```python
from build123d import *

# Parameters (mm, degrees)
PAD_DEPTH       = 30
POCKET_DEPTH    = 28
SKETCH002_R     = 1
POCKET001_DEPTH = 5
SKETCH003_R     = 1.6
POCKET002_DEPTH = 5
POCKET003_DEPTH = 2


with BuildPart() as part:
    # Sketch → Pad (new body)
    with BuildSketch(Plane.XZ):
        Polygon((-68.72, 55.88), (-68.72, -25.12), (-13.72, -25.12), (-13.72, -125.12), (22.28, -125.12), (22.28, -25.12), (77.28, -25.12), (77.28, 55.88), align=None)
    extrude(amount=PAD_DEPTH)

    # Sketch001 (on Face10 of Pad) → Pocket (cut)
    with BuildSketch(Plane.XZ.offset(30)):
        Polygon((-65.72, 52.88), (-65.72, -22.12), (-10.72, -22.12), (-10.72, -122.12), (19.28, -122.12), (19.28, -22.12), (74.28, -22.12), (74.28, 52.88), align=None)
    extrude(amount=-POCKET_DEPTH, mode=Mode.SUBTRACT)

    # Sketch002 (on Face10 of Pad) → Pocket001 (cut)
    with BuildSketch(Plane.XZ.offset(30)):
        with Locations((-11.82, -23.22)):
            Circle(SKETCH002_R)
        with Locations((-11.72, -123.12)):
            Circle(SKETCH002_R)
        with Locations((20.38, -23.22)):
            Circle(SKETCH002_R)
        with Locations((20.28, -123.12)):
            Circle(SKETCH002_R)
        with Locations((-66.72, -23.12)):
            Circle(SKETCH002_R)
        with Locations((75.28, -23.12)):
            Circle(SKETCH002_R)
        with Locations((75.28, 53.88)):
            Circle(SKETCH002_R)
        with Locations((-66.72, 53.88)):
            Circle(SKETCH002_R)
    extrude(amount=-POCKET001_DEPTH, mode=Mode.SUBTRACT)

    # Sketch003 (on Face28 of Pocket001) → Pocket002 (cut)
    with BuildSketch(Plane.XZ.offset(2)):
        with Locations((-7.62, -119.62)):
            Circle(SKETCH003_R)
        with Locations((16.78, -119.62)):
            Circle(SKETCH003_R)
        with Locations((-7.62, -26.62)):
            Circle(SKETCH003_R)
        with Locations((16.78, -26.62)):
            Circle(SKETCH003_R)
    extrude(amount=-POCKET002_DEPTH, mode=Mode.SUBTRACT)

    # Sketch004 (on Face5 of Pocket002) → Pocket003 (cut)
    with BuildSketch(Plane.XZ.offset(30)):
        Polygon((-67.97, 55.13), (-67.97, -24.37), (-12.97, -24.37), (-12.97, -124.37), (21.53, -124.37), (21.53, -24.37), (76.53, -24.37), (76.53, 55.13), align=None)
    extrude(amount=-POCKET003_DEPTH, mode=Mode.SUBTRACT)


solid = part.part
```
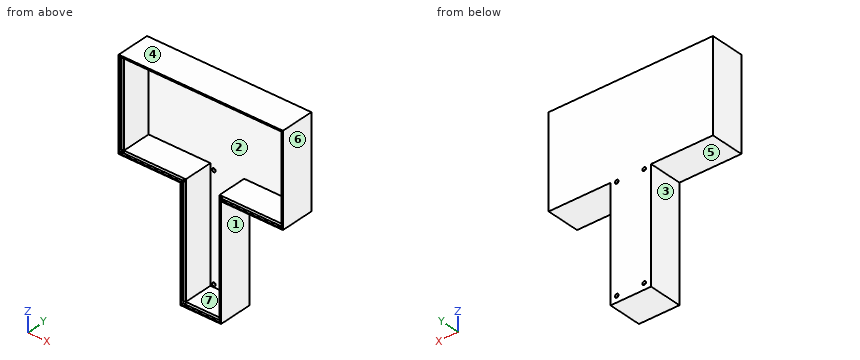
Input: part model. Units: mm. Frame: model coordinates. Face numbers are marked on the shaded views. A direction names the side the tool comes from. Coordinates: 2 decimals unless noted, no trailing zeros. Loops run counter-clockwise (first coordinate to the right, second up) from the corner with the lowest first, then second, coordinate; pieces in that order, holes last. Notation, with made-up numbers: M 78.5,-15.5 L 99.5,-15.5 A13 cw 99.5,8.5 Z; hole C -36.5,58.5 d9. An arc over 180 degrees is marked long. Use a Markdown table: item, result. Add a question column.
1) Set-up query: the marked faces 1, 2, 3 and 4. Return all of +Z, -Z, +X, -X, +Y, -Y with unobstructed straight access to the full face (end or side cutting, diameter ignored); none if empty.
2) Section B-B, the plane z = -96. Return the cut outline in (x, y).
3) Line query: L1, parallel to Z at x = -66.72, y = -27.3; L2, parallel to X at y = -25, z = -92.5; L3, parallel to Z at x = 26, y = -6. Output: solid intervals per line, ascending. Write a range as from..to.
4) Section A-A, the plane y = -16. Return the cut outline in (x, z).
5) Draft query along X for the marked faces 5, 6 and 7. Return one class per face: +X half, -X half, draft (parallel to the pull), parting line (faces both ways), or undercut.
6) Section C-C, the plane x = 26.5. Return the cut outline in (y, z), plus the area to 3 significant figures.
7) Pin query (flat end, axial travel): P1, Ø5, axis at y = -5.5, z = -89.5, coming from the -X side; P2, Ø5, axis at x = 45, y = -15.5, coming from the -Z side; P3, Ø1, axis at x = -36, z = 22, coming from the -Y side; P4, Ø1.9, axis at x = 16.78, z = -26.62, coming from the +Y side. Return the tip coordinate at first contact, or that it passes through.
Answer below:
| question | item | result |
|---|---|---|
| 1 | face 1 | -Z, +X, +Y, -Y |
| 1 | face 2 | -Y |
| 1 | face 3 | -Z, -X, +Y, -Y |
| 1 | face 4 | +Z, +X, -X, +Y, -Y |
| 2 | outline | M -13.72,-30 L -12.97,-30 L -12.97,-28 L -10.72,-28 L -10.72,-2 L 19.28,-2 L 19.28,-28 L 21.53,-28 L 21.53,-30 L 22.28,-30 L 22.28,0 L -13.72,0 Z |
| 3 | L1 | -25.12..-24.12, -22.12..52.88, 54.88..55.88 |
| 3 | L2 | -13.72..-10.72, 19.28..22.28 |
| 3 | L3 | -25.12..-22.12, 52.88..55.88 |
| 4 | outline | M -68.72,-25.12 L -13.72,-25.12 L -13.72,-125.12 L 22.28,-125.12 L 22.28,-25.12 L 77.28,-25.12 L 77.28,55.88 L -68.72,55.88 Z; hole M -65.72,-22.12 L -10.72,-22.12 L -10.72,-122.12 L 19.28,-122.12 L 19.28,-22.12 L 74.28,-22.12 L 74.28,52.88 L -65.72,52.88 Z |
| 5 | face 5 | draft |
| 5 | face 6 | +X half |
| 5 | face 7 | undercut |
| 6 | outline | M -30,-25.12 L 0,-25.12 L 0,55.88 L -30,55.88 L -30,55.13 L -28,55.13 L -28,52.88 L -2,52.88 L -2,-22.12 L -28,-22.12 L -28,-24.37 L -30,-24.37 Z |
| 6 | area | 321 mm2 |
| 7 | P1 | x = -13.72 |
| 7 | P2 | z = -25.12 |
| 7 | P3 | y = -2 |
| 7 | P4 | through |
